Could you check a few things on this model? Use its own coordinates, in mm. Face numbers are marked on the shaded views. A direction names the side the tool comes from. Coordinates: 2 decimals unless noted, no trailing zeros. Write each loop counter-clockwise with the first axis right and the second up, starting at its lowest first coordinate (ties: lowest second). Pieces come first, ordered by that corner, then holes.
Item 1: Thinking about a two-plate mould opening in X: for the marked faces 4, 5 and 6, which applies, +X half, -X half, draft (parallel to the pull), parting line (faces both ways), or undercut?
Item 2: For P1, Ø3, axis at x = 13.5, z = 51, coming from the +Y side; P2, Ø2, axis at y = 33, z = 34.5, coming from the -X side; P3, Ø15, axis at x = 84, z = 19.5, coming from the +Y side, each with a flat end and sliding along its axis, tell me the tip position at first contact or that it passes through.
Item 3: Which directions (+Z, -Z, +X, -X, +Y, -Y) give clear straight access to the entire face, cutting with the end or side of a thin tool? Please do the marked faces 1, 2 and 3.
Item 4: I want a section at B-B on z = 15.5. Please give me the cut outline in (x, y).
Item 5: I want a section at C-C on y = 35. Please give me the cut outline in (x, z), then the cut area to 3 significant figures.
Item 6: I want a section at A-A on x = 25. Please give me the cut outline in (y, z), then the cut area to 3 significant figures.
Item 7: If I drill on probe 1 along Y at (x, z) = (78, 8.5); probe 2 along Y at (x, z) = (40, 46); probe 3 along X at (y, z) = (30.5, 45.5), over which ranges is the centre line in solid material (lowest first)?
Item 8: I want a section at D-D on x = 86. Please give me the cut outline in (y, z), then the cut area to 3 significant figures.
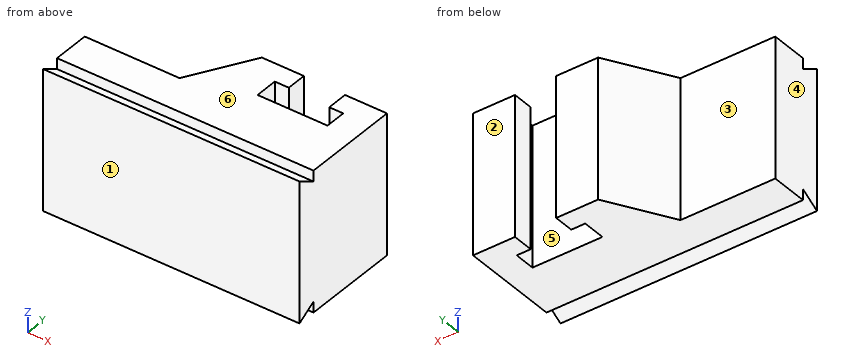
from build123d import *

# Parameters (mm, degrees)
BOSS_EXTRUDE1_DEPTH = 60
BOSS_EXTRUDE2_DEPTH = 110


with BuildPart() as part:
    # Sketch1 → Boss-Extrude1 (new body)
    with BuildSketch(Plane.XY):
        Polygon((0, 0), (110, 0), (110, 42), (92, 42), (92, 33), (98, 33), (98, 24), (68, 24), (68, 33.834738617), (74, 33.834738617), (74, 42.44856661), (56, 42.44856661), (40.640659473, 15.845408447), (0, 15.845408447), align=None)
    extrude(amount=BOSS_EXTRUDE1_DEPTH)

    # Sketch2 → Boss-Extrude2 (add)
    with BuildSketch(Plane.ZY):
        Polygon((0, -8), (60, -8), (55.381197846, 0), (4.618802154, 0), align=None)
    extrude(amount=-BOSS_EXTRUDE2_DEPTH)


solid = part.part
Response values:
1. face 4: -X half
1. face 5: undercut
1. face 6: draft
2. P1: stops at y = 15.85
2. P2: stops at x = 49.97
2. P3: stops at y = 24
3. face 1: +Z, -Z, +X, -X, -Y
3. face 2: +Z, -Z, +X, +Y
3. face 3: +Z, -Z, -X, +Y
4. outline: (0, -8) - (110, -8) - (110, 42) - (92, 42) - (92, 33) - (98, 33) - (98, 24) - (68, 24) - (68, 33.83) - (74, 33.83) - (74, 42.45) - (56, 42.45) - (40.64, 15.85) - (0, 15.85) - close
5. outline: (51.7, 0) - (74, 0) - (74, 60) - (51.7, 60) - close; (92, 0) - (110, 0) - (110, 60) - (92, 60) - close
5. area: 2,420 mm2
6. outline: (-8, 0) - (0, 4.62) - (0, 0) - (15.85, 0) - (15.85, 60) - (0, 60) - (0, 55.38) - (-8, 60) - close
6. area: 1,390 mm2
7. probe 1: y = -8 to 24
7. probe 2: y = -8 to 15.85
7. probe 3: x = 49.1 to 68, 98 to 110
8. outline: (-8, 0) - (0, 4.62) - (0, 0) - (24, 0) - (24, 60) - (0, 60) - (0, 55.38) - (-8, 60) - close
8. area: 1,880 mm2
